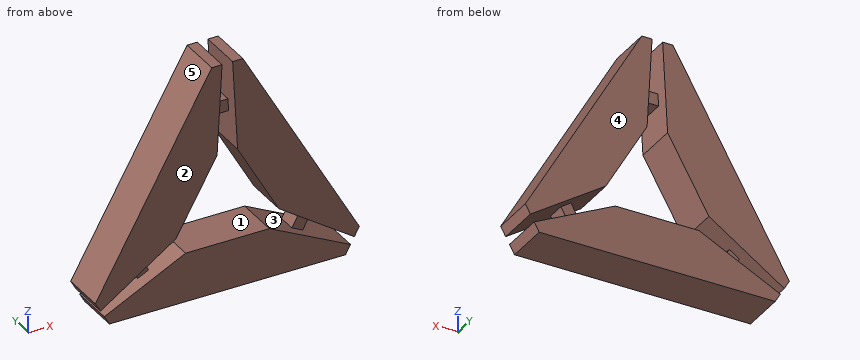
from build123d import *

# Parameters (mm, degrees)
F1_DEPTH = 3.6
F3_DEPTH = 1.5


with BuildPart() as f1:
    # F0 (on Front) → F1 (new body, symmetric)
    with BuildSketch(Plane.XZ):
        Polygon((-20.8257506798, 2.9768245619), (-8.3789686798, 11.3850395619), (-1.5652516798, 23.4041475619), (-0.7448276798, 38.3654525619), (-2.4436836798, 38.3654525619), (-21.6676586798, 4.4551755619), align=None)
    extrude(amount=F1_DEPTH, both=True)



with BuildPart() as f1b:
    # F0 (on Front) → F1, piece 2 (new body, symmetric)
    with BuildSketch(Plane.XZ):
        Polygon((1.8247563202, 23.4041475619), (8.6384733202, 11.3850395619), (21.0967113202, 2.9690845619), (21.9271633202, 4.4551755619), (2.7031873202, 38.3654525619), (1.0043313202, 38.3654525619), align=None)
    extrude(amount=F1_DEPTH, both=True)


with BuildPart() as f1c:
    # F0 (on Front) → F1, piece 3 (new body, symmetric)
    with BuildSketch(Plane.XZ):
        Polygon((7.0596503202, 8.5081085619), (-6.7564876798, 8.5081085619), (-20.1794006798, 1.8418635619), (-19.3385966798, 0.3654525619), (19.6417593202, 0.3654525619), (20.4702253202, 1.8479905619), align=None)
    extrude(amount=F1_DEPTH, both=True)


with BuildPart() as f1_1:
    add(f1.part)

    add(f1b.part)  # F3 merges F1b

    add(f1c.part)  # F3 merges F1c
    # F2 (on Front) → F3 (join, symmetric)
    with BuildSketch(Plane.XZ):
        Polygon((1.4145438202, 30.8848000619), (-1.1550396798, 30.8848000619), (-1.2647124657, 28.8848000619), (1.5242167398, 28.8848000619), align=None)
        Polygon((-12.939735993, 8.3040896316), (-14.6023596798, 7.1809320619), (-13.4679441798, 5.1749860619), (-11.6739917823, 6.0659198107), align=None)
        Polygon((11.9765909947, 6.0661994647), (13.7649378202, 5.1780495619), (14.8675923202, 7.1770620619), (13.207815063, 8.2982969193), align=None)
    extrude(amount=F3_DEPTH, both=True)


solid = f1_1.part
The model under review builds one solid part; all positions refer to its coordinate system, in mm. Face numbers are marked on the shaded views. A direction names the side the tool comes from. Round coordinates to 2 decimals unless told otherwise and drop trailing zeros. Write each loop counter-clockwise with the first axis right and the second up, starting at its lowest first coordinate (ties: lowest second). Pieces come first, ordered by that corner, then holes. Notation, with made-up numbers: M 54,-5.75 L 104,-5.75 A10 ccw 104,11.25 Z; hole C 65,-13.5 d7. An arc over 180 degrees is marked long. Answer as CSV lines item,"result". Start each with the question number.
Q1. The part is to be moulded in two halves that separate along Z. For the marked faces 3, 4 and 5, say which applies: +Z half, -Z half, draft (parallel to the pull), parting line (faces both ways), or undercut.
Q2. Consider section C-C, the plane x = -14. Give the boundary of the cut face in (y, z), then the cut area to 3 significant figures.
Q3. Tool access review of the marked faces 1 and 2: name each direction out of +Z, -Z, +X, -X, +Y, -Y from which nothing blocks a thin tool from reaching the whole face with its end or side.
Q4. Consider section A-A, the plane y = -2. Give the boundary of the cut face in (x, z).
Q5. Clearance check with flat-ended pins moving along their axes: P1, Ø0.6, axis at x = 0, z = 29.5, coming from the -Y side; P2, Ø0.9, axis at x = 13.5, z = 7.5, coming from the +Y side; P3, Ø3, axis at y = 1.5, z = 11, coming from the -X side; P4, Ø3, axis at x = 0.5, z = 11.5, coming from the +Y side. State where each tip first meets the part, or that it passes through.
Q6. Wall thickness on line 1 along X through (y, z) = (2.75, 5); line 2 along Z through (x, y) = (6, 2); line 3 along Z through (x, y) = (-10.5, 2.25): over which ranges is each line inside the solid? List them lowest first.
Q7. Consider section B-B, the plane z = 36.5. Give the boundary of the cut face in (x, y).
Q8. Consider section D-D, the plane z = 9.5. Give the boundary of the cut face in (x, y).
Result set:
1,face 3,"undercut"
1,face 4,"draft"
1,face 5,"+Z half"
2,outline,"M -3.6,0.37 L 3.6,0.37 L 3.6,4.91 L -3.6,4.91 Z; M -3.6,7.59 L -1.5,7.59 L -1.5,6.12 L 1.5,6.12 L 1.5,7.59 L 3.6,7.59 L 3.6,17.98 L -3.6,17.98 Z"
2,area,"112 mm²"
3,face 1,"+Y, -Y"
3,face 2,"+Z, -Z, +X, -X, -Y"
4,outline,"M -21.67,4.46 L -20.83,2.98 L -8.38,11.39 L -1.57,23.4 L -0.74,38.37 L -2.44,38.37 Z; M -20.18,1.84 L -19.34,0.37 L 19.64,0.37 L 20.47,1.85 L 7.06,8.51 L -6.76,8.51 Z; M 1,38.37 L 1.82,23.4 L 8.64,11.39 L 21.1,2.97 L 21.93,4.46 L 2.7,38.37 Z"
5,P1,"stops at y = -1.5"
5,P2,"stops at y = 1.5"
5,P3,"stops at x = -18.81"
5,P4,"passes through"
6,line 1,"x = -21.36 to -17.83, -13.82 to 14.12, 18.09 to 21.62"
6,line 2,"z = 0.37 to 8.51, 16.04 to 32.55"
6,line 3,"z = 0.37 to 6.65, 9.95 to 24.15"
7,outline,"M -3.5,-3.6 L -0.85,-3.6 L -0.85,3.6 L -3.5,3.6 Z; M 1.11,-3.6 L 3.76,-3.6 L 3.76,3.6 L 1.11,3.6 Z"
8,outline,"M -18.81,-3.6 L -11.17,-3.6 L -11.17,3.6 L -18.81,3.6 Z; M 11.43,-3.6 L 19.07,-3.6 L 19.07,3.6 L 11.43,3.6 Z"
